CAD build for the part. Positions are in the model's coordinates, mm. A direction names the side the tool comes from. Give positions to 0.01 mm unless a question says otherwise; leave off trailing zeros. Loops run counter-clockwise (first coordinate to the right, second up) from the corner with the lowest first, then second, coordinate; pieces in that order, holes last. Notation, with made-up numbers: M 64,35.25 L 108,35.25 A14 ccw 108,45.25 Z; hole C -18.5,-17.5 d6. An arc over 180 degrees is marked long. Answer as CSV lines item,"result".
from build123d import *

# Parameters (mm, degrees)
F0_R          = 29
F1_DEPTH      = 4
F2_R          = 26.15
F3_DEPTH      = 5
F4_SIZE       = 3.99999
F5_R          = 4
F6_DEPTH      = 25
F6_DEPTH_BACK = 25
F7_R          = 2.5
F8_DEPTH      = 25
F8_DEPTH_BACK = 25


# Not quite as in the source:
# - a fillet or chamfer is up to 0.001 mm smaller than in the source, because OpenCascade refuses the exact size


with BuildPart() as f1:
    # F0 (on Top) → F1 (new body)
    with BuildSketch(Plane.XY):
        Circle(F0_R)
    extrude(amount=F1_DEPTH)

    # F2 (on Top) → F3 (join)
    with BuildSketch(Plane.XY):
        Circle(F2_R)
    extrude(amount=-F3_DEPTH)

    # F4 (size 4 in the source; OpenCascade refuses exactly that, so slightly less here)
    f4_edges = [f1.edges().sort_by_distance(p)[0] for p in [
        (-29, 0, 4),
    ]]
    chamfer(f4_edges, length=F4_SIZE)

    # F5 (on Top) → F6 (cut, two sides)
    with BuildSketch(Plane.XY) as f6_sk:
        Circle(F5_R)
    extrude(amount=F6_DEPTH, mode=Mode.SUBTRACT)
    extrude(f6_sk.sketch, amount=-F6_DEPTH_BACK, mode=Mode.SUBTRACT)

    # F7 (on Top) → F8 (cut, two sides)
    with BuildSketch(Plane.XY) as f8_sk:
        with Locations((8.8876162109, 12.0834712764)):
            Circle(F7_R)
    extrude(amount=F8_DEPTH, mode=Mode.SUBTRACT)
    extrude(f8_sk.sketch, amount=-F8_DEPTH_BACK, mode=Mode.SUBTRACT)


solid = f1.part
1) Flat gauge pins, fed straight in: pin 1 (13 mm diameter, centred on x = 0, y = 0, fed in from -Z); pin 2 (1 mm diameter, centred on y = 10, z = 2, fed in from -X); pin 3 (1 mm diameter, centred on x = 6.5, z = 1, fed in from -Y); pin 4 (3 mm diameter, centred on x = 6, z = 3, fed in from +Y). Where does each tip first touch, or does it go through?
Answer below:
pin 1,"stops at z = -5"
pin 2,"stops at x = -25.65"
pin 3,"stops at y = -27.76"
pin 4,"stops at y = 26.87"
2) Which spindle directions (+Z, -Z, +X, -X, +Y, -Y) get a long thin tool onto all of the face, cutting with end or side? Do faces 1 (the face through (-5.669, -25.528, -2.465)), 2 (the face through (0, -5, 4)). Say none if no direction does.
Answer below:
face 1,"-Z"
face 2,"+Z, +X, -X, +Y, -Y"
3) Band-saw the part on C-C on z = -0.75. Give the cut face in (x, y).
Answer below:
outline,"C 0,0 d52.3; hole C 0,0 d8; hole C 8.89,12.08 d5"
4) Drill centre lines: line 1 (X direction, y = -1.5, z = -1.5); line 2 (X direction, y = 11, z = -4.25); line 3 (Y direction, x = 1, z = -2.5). Where is each one in solid material? Low to high. Write a range as from..to.
Answer below:
line 1,"x = -26.11..-3.71, 3.71..26.11"
line 2,"x = -23.72..6.63, 11.14..23.72"
line 3,"y = -26.13..-3.87, 3.87..26.13"
